Input: dimensioned drawing with shaded views. Units: mm. Origin: part minimum x, y, z. Give positions to 0.01 mm unless a question says otherwise; leave off trailing zeros. Loops run counter-clockwise (first coordinate to the right, second up) from the corner with the lowest first, then second, coordinate; pieces in that order, holes last.
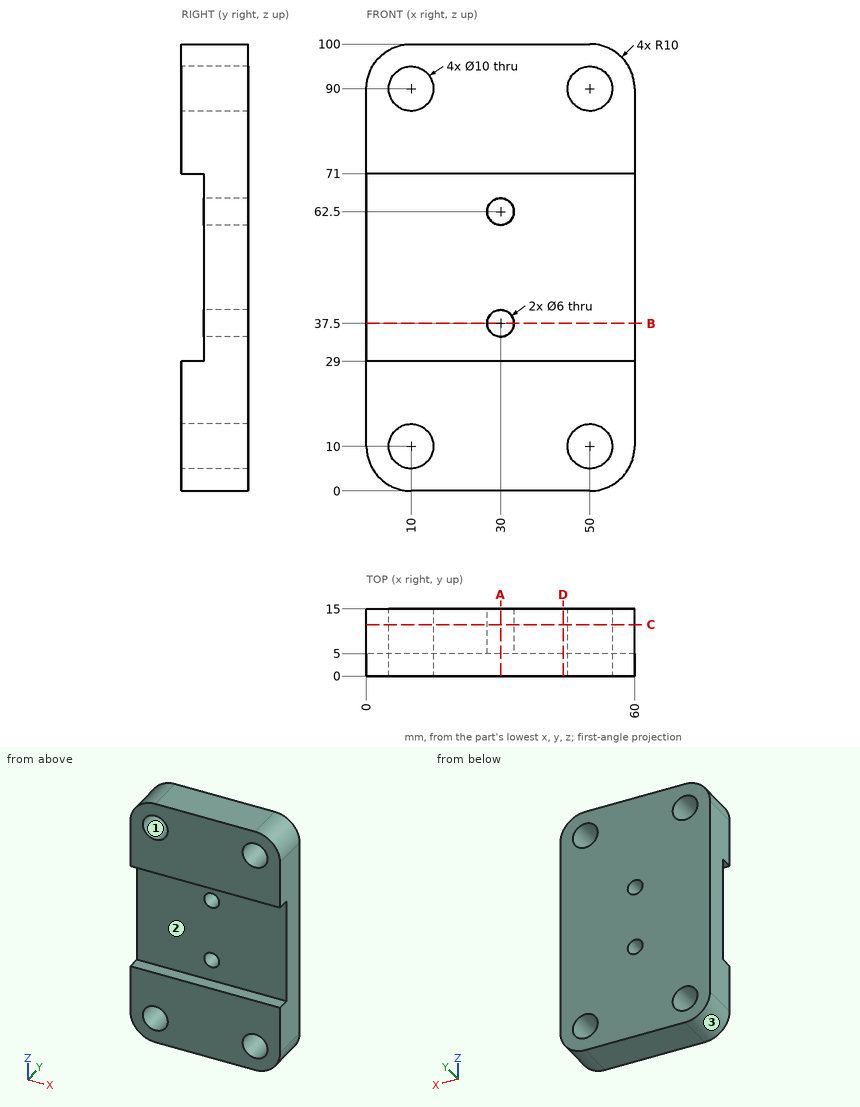
(1) First-contact query: pin 1 (7 mm diameter, centred on x = 30, z = 62.5, fed in from -Y). Flat tip, straight axial feed; report the tip coordinate or a pass-through.
A:
pin 1: stops at y = 5
(2) Section C-C, the plane y = 11.5. Return the cut outline in (x, z), then the cut area to 3 significant figures.
A:
outline: (0, 10) arc R10 ccw to (10, 0) - (50, 0) arc R10 ccw to (60, 10) - (60, 90) arc R10 ccw to (50, 100) - (10, 100) arc R10 ccw to (0, 90) - close; hole circle Ø10 at (10, 10); hole circle Ø10 at (10, 90); hole circle Ø6 at (30, 37.5); hole circle Ø6 at (30, 62.5); hole circle Ø10 at (50, 10); hole circle Ø10 at (50, 90)
area: 5,540 mm2
(3) Section B-B, the plane z = 37.5. Return the cut outline in (x, y), then the cut area to 3 significant figures.
A:
outline: (0, 5) - (27, 5) - (27, 15) - (0, 15) - close; (33, 5) - (60, 5) - (60, 15) - (33, 15) - close
area: 540 mm2
(4) Mould query, pull axis X, two halves, no side actions, for the marked faces 1, 2 and 3. Classes: pulls with the +X half, pulls with the -X half, needs draft (parallel to the pull), parting line crosses it, or undercut.
A:
face 1: undercut
face 2: needs draft
face 3: pulls with the -X half
(5) Section A-A, the plane x = 30. Return the cut outline in (y, z), then the cut area to 3 significant figures.
A:
outline: (0, 0) - (15, 0) - (15, 34.5) - (5, 34.5) - (5, 29) - (0, 29) - close; (0, 71) - (5, 71) - (5, 65.5) - (15, 65.5) - (15, 100) - (0, 100) - close; (5, 40.5) - (15, 40.5) - (15, 59.5) - (5, 59.5) - close
area: 1,170 mm2
(6) Ray query, line 1 along Z through (x, y) = (50, 9); line 2 along Z through (x, y) = (30, 8.5); line 3 along Z through (x, y) = (10, 3.5). Return the intervals inside material, ascending.
A:
line 1: z = 0 to 5, 15 to 85, 95 to 100
line 2: z = 0 to 34.5, 40.5 to 59.5, 65.5 to 100
line 3: z = 0 to 5, 15 to 29, 71 to 85, 95 to 100
(7) Section D-D, the plane x = 44. Return the cut outline in (y, z).
A:
outline: (0, 0) - (15, 0) - (15, 100) - (0, 100) - (0, 71) - (5, 71) - (5, 29) - (0, 29) - close
